```python
from build123d import *

# Parameters (mm, degrees)
F0_W     = 93
F0_H     = 64
F1_DEPTH = 18
F2_T     = -1.5
F3_R     = 2.25
F3_R_2   = 1.25
F4_DEPTH = 6
F5_DEPTH = 4.5
F3_R_3   = 1.6
F6_DEPTH = 13


with BuildPart() as f1:
    # F0 (on Top) → F1 (new body)
    with BuildSketch(Plane.XY):
        Rectangle(F0_W, F0_H)
    extrude(amount=F1_DEPTH)

    # F2
    f2_openings = [f1.faces().sort_by_distance(p)[0] for p in [
        (0, 0, 18),
    ]]
    offset(amount=F2_T, openings=f2_openings)

    # F3 (on Top) → F4 (join)
    with BuildSketch(Plane.XY):
        with Locations((-29.5, -14.25)):
            Circle(F3_R)
        with Locations((-29.5, -14.25)):
            Circle(F3_R_2, mode=Mode.SUBTRACT)
        with Locations((24.5, -14.25)):
            Circle(F3_R)
        with Locations((24.5, -14.25)):
            Circle(F3_R_2, mode=Mode.SUBTRACT)
        with Locations((24.5, 13.75)):
            Circle(F3_R)
        with Locations((24.5, 13.75)):
            Circle(F3_R_2, mode=Mode.SUBTRACT)
    extrude(amount=F4_DEPTH)

    # F3 (on Top) → F5 (join)
    with BuildSketch(Plane.XY):
        with Locations((-29.5, 13.75)):
            Circle(F3_R)
        with Locations((-29.5, 13.75)):
            Circle(F3_R_2, mode=Mode.SUBTRACT)
    extrude(amount=F5_DEPTH)

    # F3 (on Top) → F6 (join)
    with BuildSketch(Plane.XY):
        with BuildLine():
            Line((-19.85, 31), (-26.35, 31))
            Line((-26.35, 31), (-26.35, 26))
            ThreePointArc((-26.35, 26), (-23.1, 22.75), (-19.85, 26))
            Line((-19.85, 26), (-19.85, 31))
        make_face()
        with Locations((-23.1, 26)):
            Circle(F3_R_3, mode=Mode.SUBTRACT)
        with BuildLine():
            Line((21.075, 31), (14.575, 31))
            Line((14.575, 31), (14.575, 26))
            ThreePointArc((14.575, 26), (17.825, 22.75), (21.075, 26))
            Line((21.075, 26), (21.075, 31))
        make_face()
        with Locations((17.825, 26)):
            Circle(F3_R_3, mode=Mode.SUBTRACT)
        with BuildLine():
            Line((14.575, -26), (14.575, -31))
            Line((14.575, -31), (21.075, -31))
            Line((21.075, -31), (21.075, -26))
            ThreePointArc((21.075, -26), (17.825, -22.75), (14.575, -26))
        make_face()
        with Locations((17.825, -26)):
            Circle(F3_R_3, mode=Mode.SUBTRACT)
        with BuildLine():
            Line((-26.35, -26), (-26.35, -31))
            Line((-26.35, -31), (-19.85, -31))
            Line((-19.85, -31), (-19.85, -26))
            ThreePointArc((-19.85, -26), (-23.1, -22.75), (-26.35, -26))
        make_face()
        with Locations((-23.1, -26)):
            Circle(F3_R_3, mode=Mode.SUBTRACT)
    extrude(amount=F6_DEPTH)


solid = f1.part
```
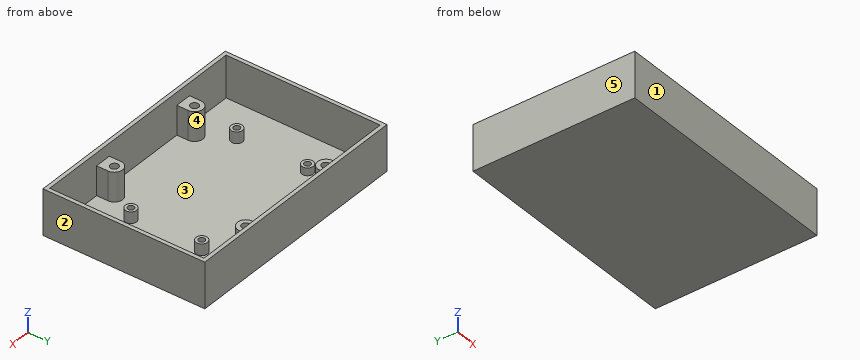
Verification items for the finished model (mm, model axes). Face numbers are marked on the shaded views. A direction names the side the tool comes from. Give positions to 0.01 mm unless a question says otherwise; leave off trailing zeros. Order: outer loops, then holes, each group sorted by start corner. A loop starts at its lowest first (then second) coordinate and runs counter-clockwise, first axis right, second up. Notation, with made-up numbers: M -6,-30.75 L 6,-30.75 A12 ccw 6,-21.75 Z; hole C -11.5,13.5 d1. An arc over 180 degrees is marked long. Answer in a Markdown table with one row per item. Add a question column.
Item 1: Tool access check on the marked faces 4 and 5. Record the directions out of +Z, -Z, +X, -X, +Y, -Y that give a thin tool (end or side, any length) a straight path to the whole face; none if there is none.
Item 2: Section check C-C, the plane y = -14.25. Enter the section's corners in (x, z), and give its area (3 significant figures).
Item 3: Gauge pin test, flat ends, axial feed: pin 1 (3 mm diameter, centred on x = -29.5, y = -14.25, fed in from +Z); pin 2 (5 mm diameter, centred on x = 19, y = 25.5, fed in from +Z); pin 3 (5 mm diameter, centred on x = 11.5, y = 16, fed in from +Z). Record the tip position at first contact, or that the pin passes through.
Item 4: Section check B-B, the plane x = -23.1. Enter the section's corners in (y, z).
Item 5: Section check A-A, the plane z = 15.25. Enter the section's corners in (x, y), and give its area (3 significant figures).
Item 6: Scan lines: probe 1 along X at (y, z) = (-26, 8.25) (3 decimals); probe 2 along Y at (x, z) = (-23.1, 10.75). Record each from-to range of solid material in increasing order. Write a range as from..to.
Item 7: Mould release check, pull along X, two halves, no side actions. Record for the marked faces 1, 2 and 3: released by +X, released by -X, zero draft, split by the parting line, or undercut.
Item 8: Section check D-D, the plane z = 8.25. Enter the section's corners in (x, y) (3 decimals), and give its area (3 significant figures).
Filled sheet:
| question | item | result |
|---|---|---|
| 1 | face 4 | +Z |
| 1 | face 5 | +Z, -Z, -X, +Y, -Y |
| 2 | outline | M -46.5,0 L 46.5,0 L 46.5,18 L 45,18 L 45,1.5 L 26.75,1.5 L 26.75,6 L 25.75,6 L 25.75,1.5 L 23.25,1.5 L 23.25,6 L 22.25,6 L 22.25,1.5 L -27.25,1.5 L -27.25,6 L -28.25,6 L -28.25,1.5 L -30.75,1.5 L -30.75,6 L -31.75,6 L -31.75,1.5 L -45,1.5 L -45,18 L -46.5,18 Z |
| 2 | area | 207 mm^2 |
| 3 | pin 1 | stops at z = 6 |
| 3 | pin 2 | stops at z = 13 |
| 3 | pin 3 | stops at z = 1.5 |
| 4 | outline | M -32,0 L 32,0 L 32,18 L 30.5,18 L 30.5,13 L 27.6,13 L 27.6,1.5 L 24.4,1.5 L 24.4,13 L 22.75,13 L 22.75,1.5 L -22.75,1.5 L -22.75,13 L -24.4,13 L -24.4,1.5 L -27.6,1.5 L -27.6,13 L -30.5,13 L -30.5,18 L -32,18 Z |
| 5 | outline | M -46.5,-32 L 46.5,-32 L 46.5,32 L -46.5,32 Z; hole M -45,-30.5 L 45,-30.5 L 45,30.5 L -45,30.5 Z |
| 5 | area | 462 mm^2 |
| 6 | probe 1 | x = -46.5..-45, -26.35..-24.7, -21.5..-19.85, 14.575..16.225, 19.425..21.075, 45..46.5 |
| 6 | probe 2 | y = -32..-27.6, -24.4..-22.75, 22.75..24.4, 27.6..32 |
| 7 | face 1 | zero draft |
| 7 | face 2 | released by +X |
| 7 | face 3 | undercut |
| 8 | outline | M -46.5,-32 L 46.5,-32 L 46.5,32 L -46.5,32 Z; hole M -45,-30.5 L -26.35,-30.5 L -26.35,-26 A3.25 cw -19.85,-26 L -19.85,-30.5 L 14.575,-30.5 L 14.575,-26 A3.25 cw 21.075,-26 L 21.075,-30.5 L 45,-30.5 L 45,30.5 L 21.075,30.5 L 21.075,26 A3.25 cw 14.575,26 L 14.575,30.5 L -19.85,30.5 L -19.85,26 A3.25 cw -26.35,26 L -26.35,30.5 L -45,30.5 Z; hole C -23.1,-26 d3.2; hole C -23.1,26 d3.2; hole C 17.825,-26 d3.2; hole C 17.825,26 d3.2 |
| 8 | area | 613 mm^2 |
